```python
from build123d import *

# Parameters (mm, degrees)
SKETCH_1_W          = 134
SKETCH_1_H          = 72
EXTRUDE_1_DEPTH     = 3
SKETCH_2_W          = 58
SKETCH_2_H          = 62
CUT_EXTRUDE_1_DEPTH = 77.118328936
SKETCH_2_4_W        = 58
SKETCH_2_4_H        = 2
EXTRUDE_2_DEPTH     = 2
EXTRUDE_3_DEPTH     = 3
SKETCH_3_W          = 54
SKETCH_3_H          = 1.5
CUT_EXTRUDE_2_DEPTH = 3
SKETCH_4_R          = 0.35
CUT_EXTRUDE_3_DEPTH = 1.5
CUT_EXTRUDE_START   = -70.5
SKETCH_4_3_R        = 0.35
CUT_EXTRUDE_4_DEPTH = 1.5
SKETCH_5_R          = 0.35
CUT_EXTRUDE_5_DEPTH = 1.5
CUT_EXTRUDE_START_2 = -132.5
SKETCH_5_3_R        = 0.35
CUT_EXTRUDE_6_DEPTH = 1.5


with BuildPart() as part:
    # 草图1 → 凸台-拉伸1 (new body)
    with BuildSketch(Plane.XY):
        Rectangle(SKETCH_1_W, SKETCH_1_H)
    extrude(amount=EXTRUDE_1_DEPTH)

    # 草图2 → 切除-拉伸1 (cut, through all)
    with BuildSketch(Plane.XY.offset(3)):
        with Locations((0, -5)):
            Rectangle(SKETCH_2_W, SKETCH_2_H)
    extrude(amount=-CUT_EXTRUDE_1_DEPTH, mode=Mode.SUBTRACT)

    # 草图2<4> → 凸台-拉伸2 (add)
    with BuildSketch(Plane.XY.offset(3)):
        Polygon((-29, -36), (-29, 26), (-29, 28), (-31, 28), (-31, -36), align=None)
        with Locations((0, 27)):
            Rectangle(SKETCH_2_4_W, SKETCH_2_4_H)
        Polygon((29, 28), (29, 26), (29, -36), (31, -36), (31, 28), align=None)
    extrude(amount=EXTRUDE_2_DEPTH)

    # 草图2<5> → 凸台-拉伸3 (add)
    with BuildSketch(Plane.XY.offset(3)):
        Polygon((29, 26), (-29, 26), (-29, -36), (-27, -36), (-27, 24), (27, 24), (27, -36), (29, -36), align=None)
    extrude(amount=-EXTRUDE_3_DEPTH)

    # 草图3 → 切除-拉伸2 (cut)
    with BuildSketch(Plane.XZ.offset(-24)):
        with Locations((0, 2.25)):
            Rectangle(SKETCH_3_W, SKETCH_3_H)
    extrude(amount=-CUT_EXTRUDE_2_DEPTH, mode=Mode.SUBTRACT)

    # 草图4 → 切除-拉伸3 (cut)
    with BuildSketch(Plane.XZ.offset(36)):
        with Locations(Location((-37, 1.5, 0), (0, 0, 270))):
            Circle(SKETCH_4_R)
        with Locations(Location((37, 1.5, 0), (0, 0, 270))):
            Circle(SKETCH_4_R)
    extrude(amount=-CUT_EXTRUDE_3_DEPTH, mode=Mode.SUBTRACT)

    # 草图4<3> → 切除-拉伸4 (cut)
    with BuildSketch(Plane.XZ.offset(36).offset(CUT_EXTRUDE_START)):
        with Locations(Location((-37, 1.5, 0), (0, 0, 270))):
            Circle(SKETCH_4_3_R)
        with Locations(Location((37, 1.5, 0), (0, 0, 270))):
            Circle(SKETCH_4_3_R)
    extrude(amount=-CUT_EXTRUDE_4_DEPTH, mode=Mode.SUBTRACT)

    # 草图5 → 切除-拉伸5 (cut)
    with BuildSketch(Plane(origin=(67, 0, 0), x_dir=(0, 0, -1), z_dir=(1, 0, 0))):
        with Locations((-1.5, 16)):
            Circle(SKETCH_5_R)
        with Locations((-1.5, -16)):
            Circle(SKETCH_5_R)
    extrude(amount=-CUT_EXTRUDE_5_DEPTH, mode=Mode.SUBTRACT)

    # 草图5<3> → 切除-拉伸6 (cut)
    with BuildSketch(Plane(origin=(67, 0, 0), x_dir=(0, 0, -1), z_dir=(1, 0, 0)).offset(CUT_EXTRUDE_START_2)):
        with Locations((-1.5, 16)):
            Circle(SKETCH_5_3_R)
        with Locations((-1.5, -16)):
            Circle(SKETCH_5_3_R)
    extrude(amount=-CUT_EXTRUDE_6_DEPTH, mode=Mode.SUBTRACT)


solid = part.part
```
Geometry check sheet. Reference: the model listing, model coordinates, mm. Give positions to 0.01 mm unless a question says otherwise; leave off trailing zeros. Order: outer loops, then holes, each group sorted by start corner. A loop starts at its lowest first (then second) coordinate and runs counter-clockwise, first axis right, second up. Notation, with made-up numbers: (-27.75, 56.5) - (22.25, 56.5) arc R22 cw to (22.25, 85.5) - close; hole circle Ø5 at (-23.5, 56). An arc over 180 degrees is marked (long way). Write item = value, one per line. Start each with the question number.
1) Section check C-C (x = -55). Enter the section's corners in (y, z).
2) Draft check along X on faces 1 (the flat face through (67, -1, 1)), 2 (the flat face through (0, 25, 1.5)), 3 (the flat face through (-1, 33, 3)), 4 (the flat face through (-27, -5, 2)). Enter one of: released by +X, released by -X, zero draft, split by the parting line, or undercut.
3) Scan lines: L1, parallel to Y at x = -66.4, z = 1.5; L2, parallel to X at y = -35.1, z = 1.5; L3, parallel to X at y = 35.6, z = 1.5. Record each from-to range of solid material in increasing order.
4) Section check B-B (y = 1.5). Enter the section's corners in (x, z), then the cut area to 3 significant figures.
5) Section check A-A (x = -17.5). Enter the section's corners in (y, z).
6) Gauge pin test, flat ends, axial feed: pin 1 Ø1.2 at (x, z) = (3.5, 2) entering from -Y; pin 2 Ø2 at (x, y) = (-34.5, 28) entering from -Z; pin 3 Ø0.6 at (y, z) = (-10.5, 3.5) entering from -X; pin 4 Ø8 at (x, y) = (-53.5, -1.5) entering from +Z. Record the tip position at first contact, or that the pin passes through.
Geometry check:
q1.outline = (-36, 0) - (36, 0) - (36, 3) - (-36, 3) - close
q2.face_1 = released by +X
q2.face_2 = undercut
q2.face_3 = zero draft
q2.face_4 = undercut
q3.L1 = -36 to -16.35, -15.65 to 15.65, 16.35 to 36
q3.L2 = -67 to -37.35, -36.65 to -27, 27 to 36.65, 37.35 to 67
q3.L3 = -67 to -37.35, -36.65 to 36.65, 37.35 to 67
q4.outline = (-67, 0) - (-27, 0) - (-27, 3) - (-29, 3) - (-29, 5) - (-31, 5) - (-31, 3) - (-67, 3) - close; (27, 0) - (67, 0) - (67, 3) - (31, 3) - (31, 5) - (29, 5) - (29, 3) - (27, 3) - close
q4.area = 248 mm2
q5.outline = (24, 0) - (36, 0) - (36, 3) - (28, 3) - (28, 5) - (26, 5) - (26, 3) - (27, 3) - (27, 1.5) - (24, 1.5) - close
q6.pin_1 = 24
q6.pin_2 = 0
q6.pin_3 = -31
q6.pin_4 = 3
